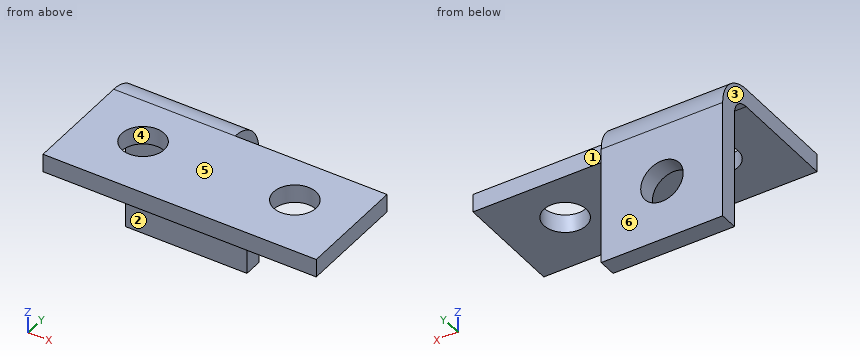
from build123d import *

# Parameters (mm, degrees)
BOSS_EXTRUDE1_DEPTH            = 40
CUT_EXTRUDE1_DEPTH             = 41
SKETCH3_W                      = 6
SKETCH3_H                      = 36
BOSS_EXTRUDE2_DEPTH            = 50
F_14_0_14_DIAMETER_HOLE1_D     = 14
F_14_0_14_DIAMETER_HOLE1_DEPTH = 51
F_14_0_14_DIAMETER_HOLE2_D     = 14
F_14_0_14_DIAMETER_HOLE2_DEPTH = 6
F_14_0_14_DIAMETER_HOLE3_D     = 14
F_14_0_14_DIAMETER_HOLE3_DEPTH = 6


with BuildPart() as part:
    # Sketch1 → Boss-Extrude1 (new body)
    with BuildSketch(Plane(origin=(-50, 0, 0), x_dir=(0, 0, -1), z_dir=(1, 0, 0))):
        with BuildLine():
            Line((0, 0), (51, 0))
            Line((51, 0), (51, 48))
            Line((51, 48), (12, 48))
            ThreePointArc((12, 48), (3.514718626, 44.485281374), (0, 36))
            Line((0, 36), (0, 0))
        make_face()
    extrude(amount=-BOSS_EXTRUDE1_DEPTH)

    # Sketch2 → Cut-Extrude1 (cut, through all)
    with BuildSketch(Plane.ZY.offset(90)):
        with BuildLine():
            Line((-51, 0), (-6, 0))
            Line((-6, 0), (-6, 36))
            ThreePointArc((-6, 36), (-7.757359313, 40.242640687), (-12, 42))
            Line((-12, 42), (-51, 42))
            Line((-51, 42), (-51, 0))
        make_face()
    extrude(amount=-CUT_EXTRUDE1_DEPTH, mode=Mode.SUBTRACT)

    # Sketch3 → Boss-Extrude2 (add)
    with BuildSketch(Plane(origin=(-50, 0, 0), x_dir=(0, 0, -1), z_dir=(1, 0, 0))):
        with Locations((3, 18)):
            Rectangle(SKETCH3_W, SKETCH3_H)
    extrude(amount=BOSS_EXTRUDE2_DEPTH)

    # Ø14.0 (14) Diameter Hole1
    with Locations(Plane.XY):
        with Locations((-70, 20)):
            Hole(F_14_0_14_DIAMETER_HOLE1_D / 2, depth=F_14_0_14_DIAMETER_HOLE1_DEPTH)

    # Ø14.0 (14) Diameter Hole2
    with Locations(Plane(origin=(0, 0, -6), x_dir=(-1, 0, 0), z_dir=(0, 0, -1))):
        with Locations((20, 20)):
            Hole(F_14_0_14_DIAMETER_HOLE2_D / 2, depth=F_14_0_14_DIAMETER_HOLE2_DEPTH)

    # Ø14.0 (14) Diameter Hole3
    with Locations(Plane(origin=(0, 42, 0), x_dir=(-1, 0, 0), z_dir=(0, -1, 0))):
        with Locations((70, 31)):
            Hole(F_14_0_14_DIAMETER_HOLE3_D / 2, depth=F_14_0_14_DIAMETER_HOLE3_DEPTH)


solid = part.part
For this review, take the finished solid that the model builds, in its own axes (mm). Face numbers are marked on the shaded views. A direction names the side the tool comes from. Round coordinates to 2 decimals unless told otherwise and drop trailing zeros. Order: outer loops, then holes, each group sorted by start corner. A loop starts at its lowest first (then second) coordinate and runs counter-clockwise, first axis right, second up. Notation, with made-up numbers: (-27, 28) -> (-23, 28) arc R23 ccw to (-23, 62) -> close; hole circle Ø6 at (28.25, -24). An arc over 180 degrees is marked (long way). Put each result on its own line as item: value.
Q1. Add section D-D on y = 14. Write out the cut boundary in (x, z).
Check result:
outline: (-90, -6) -> (-73.61, -6) -> (-73.61, 0) -> (-90, 0) -> close; (-66.39, -6) -> (-23.61, -6) -> (-23.61, 0) -> (-66.39, 0) -> close; (-16.39, -6) -> (0, -6) -> (0, 0) -> (-16.39, 0) -> close
Q2. Add section B-B on z = -31. Write out the cut boundary in (x, y).
Check result:
outline: (-90, 42) -> (-77, 42) -> (-77, 48) -> (-90, 48) -> close; (-63, 42) -> (-50, 42) -> (-50, 48) -> (-63, 48) -> close
Q3. Insertion check: pin 1 Ø11.5 at (x, z) = (-63, -23) entering from -Y; pin 2 Ø3 at (x, z) = (-31.5, -4) entering from +Y; pin 3 Ø6 at (x, y) = (-76.5, 22) entering from -Z. Each pin has a flat end and moves straight along its axis. Give the tip position at first contact, or say it passes through.
Check result:
pin 1: y = 42
pin 2: y = 36
pin 3: z = -6
Q4. Mouldability with a two-part tool opening along Y and no side actions: class the marked faces 4, 5 and 6 as pulls with the +Y half, pulls with the -Y half, needs draft (parallel to the pull), parting line crosses it, or undercut.
Check result:
face 4: undercut
face 5: needs draft
face 6: pulls with the +Y half
Q5. For probe 1 along X at (y, z) = (44.4, -31); probe 2 along Y at (x, z) = (-20, -3); probe 3 along Y at (x, z) = (-85, -14), list the stretches that pass through material, from the lowest coordinate up. Write a range as [from, to].
Check result:
probe 1: [-90, -77], [-63, -50]
probe 2: [0, 13], [27, 36]
probe 3: [42, 48]
Q6. Machinability: for the marked faces 1, 2 and 3, which of the approach directions +Z, -Z, +X, -X, +Y, -Y give a long, thin tool a straight path to every point of the face, cutting with its end or side? Answer none if there is none.
Check result:
face 1: +Z, -Z, +X, +Y
face 2: -Z, +X, -X, -Y
face 3: +Z, -Z, -X, +Y, -Y
Q7. Add section C-C on x = -20. Write out the cut boundary in (y, z).
Check result:
outline: (0, -6) -> (13, -6) -> (13, 0) -> (0, 0) -> close; (27, -6) -> (36, -6) -> (36, 0) -> (27, 0) -> close
Q8. Add section A-A on x = -70. Write out the cut boundary in (y, z).
Check result:
outline: (0, -6) -> (13, -6) -> (13, 0) -> (0, 0) -> close; (27, -6) -> (36, -6) arc R6 cw to (42, -12) -> (42, -24) -> (48, -24) -> (48, -12) arc R12 ccw to (36, 0) -> (27, 0) -> close; (42, -51) -> (48, -51) -> (48, -38) -> (42, -38) -> close
